Answer from the drawing. Dimensions are ordinates in mm from the lowest x, y and z of the part. Give positions to 0.01 mm unless a question says otherwise; leave off trailing zeros. Loops run counter-clockwise (first coordinate to the right, second up) from the corner with the lowest first, then second, coordinate; pieces in that order, holes last. Notation, with made-up numbers: M -27.75,79.5 L 13.25,79.5 A33 ccw 13.25,115.5 Z; hole C 48.5,70.5 d11. An arc over 180 degrees is marked long. Return JSON: item names as keys, results as strings. Group by question number.
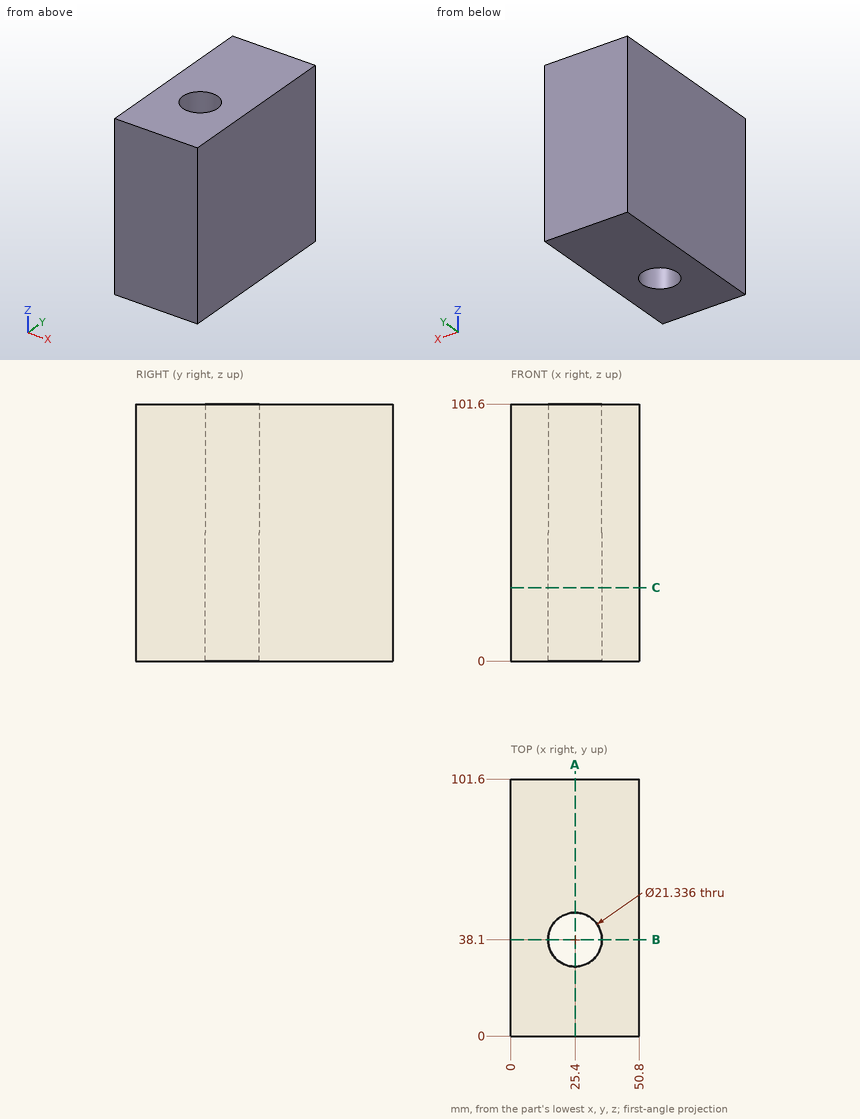
1. Straight lines are drawn through the part: line 1 along Y through (x, z) = (25.4, 16); line 2 along X through (y, z) = (37.5, 57); line 3 along X through (y, z) = (32, 92.5). For each, find the intervals that lie inside material, in ascending order.
2. Find section C-C (z = 29). Write down the section's boundary in (x, y), and give its area (3 significant figures).
3. Find section B-B (y = 38.1). Write down the section's boundary in (x, z).
4. A flat-ended cylindrical pin translates along its axis: P1, Ø13, axis at x = 25.4, y = 38.1, coming from the +Z side. Find the tip coordinate at first contact, or state that the pin passes through.
5. Find section A-A (x = 25.4). Write down the section's boundary in (y, z).
Result:
{
 "1": {"line 1": "y = 0 to 27.43, 48.77 to 101.6", "line 2": "x = 0 to 14.75, 36.05 to 50.8", "line 3": "x = 0 to 16.65, 34.15 to 50.8"},
 "2": {"outline": "M 0,0 L 50.8,0 L 50.8,101.6 L 0,101.6 Z; hole C 25.4,38.1 d21.34", "area": "4,800 mm2"},
 "3": {"outline": "M 0,0 L 14.73,0 L 14.73,101.6 L 0,101.6 Z; M 36.07,0 L 50.8,0 L 50.8,101.6 L 36.07,101.6 Z"},
 "4": {"P1": "passes through"},
 "5": {"outline": "M 0,0 L 27.43,0 L 27.43,101.6 L 0,101.6 Z; M 48.77,0 L 101.6,0 L 101.6,101.6 L 48.77,101.6 Z"}
}
